Autodesk Inventor part; units mm, degrees
ref_plane "YZ Plane" through (0, 0, 0) normal (1, 0, 0) x (0, 1, 0)
ref_plane "XZ Plane" through (0, 0, 0) normal (0, 1, 0) x (-1, 0, 0)
ref_plane "XY Plane" through (0, 0, 0) normal (0, 0, 1) x (1, 0, 0)
sketch "Sketch1" plane through (0, 0, 0) normal (0, 0, 1) x (1, 0, 0)
  circle A0 centre (0, 0) radius 3.8862
  line L0 (-19.05, 6.35) -> (19.05, 6.35)
  line L1 (19.05, 6.35) -> (19.05, -6.35)
  line L2 (19.05, -6.35) -> (-19.05, -6.35)
  line L3 (-19.05, -6.35) -> (-19.05, 6.35)
  point P0 (0, 0)
  dimension "d0" = 38.1
  dimension "d2" = 12.7
  dimension "d3" = 6.35
  dimension "d4" = 19.05
extrude "Extrusion1" add sketch "Sketch1" against normal blind 12.7
sketch "Sketch2" plane through (-19.05, 6.35, 0) normal (0, 1, 0) x (1, 0, 0)
  line L0 (38.1, 0) -> (38.1, 12.7)
  line L1 (0, 0) -> (0, 12.7)
  circle A0 centre (6.35, 6.35) radius 1.5875
  circle A1 centre (31.75, 6.35) radius 1.5875
  point P0 (19.05, 0)
  dimension "d7" = 3.175
  dimension "d9" = 6.35
  dimension "d10" = 6.35
extrude "Extrusion2" cut sketch "Sketch2" against normal up to next
fillet "Fillet1" radius 6.35 4 edges at (19.05, 0, -12.7) (19.05, 0, 0) (-19.05, 0, -12.7) (-19.05, 0, 0)
properties part number "motormount" material "ABS Plastic"
Verification items for the finished model (mm, model axes). Round coordinates to 2 decimals unless told otherwise and drop trailing zeros. Order: outer loops, then holes, each group sorted by start corner. A loop starts at its lowest first (then second) coordinate and runs counter-clockwise, first axis right, second up. Notation, with made-up numbers: (18, 86.5) -> (27, 86.5) arc R3 cw to (27, 90.5) -> close; hole circle Ø1 at (11, -37). An arc over 180 degrees is marked (long way). Put each result on its own line as item: value. Start each with the question number.
(1) Material ranges on line 1 along Y through (x, z) = (0, -2.75); line 2 along Z through (x, y) = (-12.7, 0.75); line 3 along X through (y, z) = (4, -7), recorded low to high.
(2) Section check A-A (y = 0). State how many separate pieces and enclosed holes the cut face has, then the cut area to 3 significant figures.
(3) Section check C-C (x = 0). Enter the section's corners in (y, z).
(4) Section check B-B (z = -5.75). Enter the section's corners in (x, y), then the cut area to 3 significant figures.
(5) Depth check by flat-ended pin: pin 1 Ø4 at (x, y) = (-15, 2.5) entering from +Z. Enter the tip coordinate at first touch or a pass-through.
(6) Draft check along X on faces 1 (the face through (-17.24, 0.09, -1.91)), 2 (the face through (0, -6.35, -6)), 3 (the face through (-11.234, 0.089, -5.742)), 4 (the face through (3.707, 1.167, -6.261)). Enter one of: +X half, -X half, draft (parallel to the pull), parting line (faces both ways), or undercut.
Completed:
1. line 1: y = -6.35 to -3.89, 3.89 to 6.35
1. line 2: z = -12.7 to -7.94, -4.76 to 0
1. line 3: x = -19.02 to -14.15, -11.25 to 11.25, 14.15 to 19.02
2. separate pieces: 2
2. enclosed holes: 2
2. area: 335 mm2
3. outline: (-6.35, -12.7) -> (-3.89, -12.7) -> (-3.89, 0) -> (-6.35, 0) -> close; (3.89, -12.7) -> (6.35, -12.7) -> (6.35, 0) -> (3.89, 0) -> close
4. outline: (-19.02, -6.35) -> (-14.17, -6.35) -> (-14.17, 6.35) -> (-19.02, 6.35) -> close; (-11.23, -6.35) -> (11.23, -6.35) -> (11.23, 6.35) -> (-11.23, 6.35) -> close; (14.17, -6.35) -> (19.02, -6.35) -> (19.02, 6.35) -> (14.17, 6.35) -> close; hole circle Ø7.77 at (0, 0)
4. area: 361 mm2
5. pin 1: stops at z = -0.01
6. face 1: -X half
6. face 2: draft
6. face 3: undercut
6. face 4: undercut
